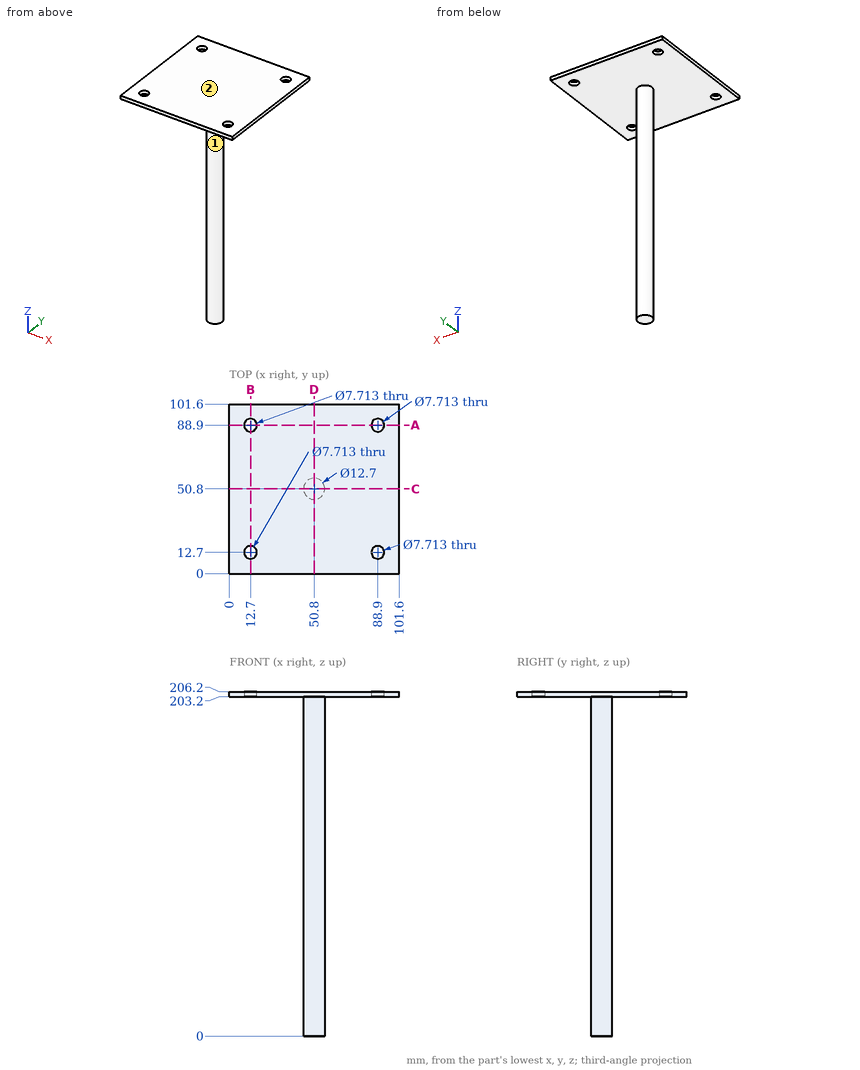
Input: dimensioned drawing with shaded views. Units: mm. Origin: part minimum x, y, z. Round coordinates to 2 decimals unless told otherwise and drop trailing zeros. Order: outer loops, then holes, each group sorted by start corner. A loop starts at its lowest first (then second) coordinate and runs counter-clockwise, first axis right, second up. Notation, with made-up numbers: (37, 22.25) -> (47, 22.25) arc R30 cw to (47, 49.25) -> close; hole circle Ø9 at (45.25, -18). An arc over 180 degrees is marked (long way). One line per item, written item: value. Start each with the question number.
Q1. Material intervals for probe 1 along Y at (x, z) = (12.7, 203.95); probe 2 along Y at (x, z) = (88, 204), sorted ascending.
Q2. Draft query along X for the marked faces 1 and 2. Return one class per face: pulls with the +X half, pulls with the -X half, needs draft (parallel to the pull), parting line crosses it, or undercut.
Q3. Section query A-A (y = 88.9). Return the cut outline in (x, z).
Q4. Section query C-C (y = 50.8). Return the cut outline in (x, z), plus the area to 3 significant figures.
Q5. Pin query (flat end, axial travel): pin 1 (3 mm diameter, centred on x = 77.5, y = 38.5, fed in from -Z); pin 2 (4.5 mm diameter, centred on x = 12.7, y = 12.7, fed in from +Z). Return the tip coordinate at first contact, or that it passes through.
Findings below:
1. probe 1: 0 to 8.84, 16.56 to 85.04, 92.76 to 101.6
1. probe 2: 0 to 8.95, 16.45 to 85.15, 92.65 to 101.6
2. face 1: parting line crosses it
2. face 2: needs draft
3. outline: (0, 203.2) -> (8.84, 203.2) -> (8.84, 206.2) -> (0, 206.2) -> close; (16.56, 203.2) -> (85.04, 203.2) -> (85.04, 206.2) -> (16.56, 206.2) -> close; (92.76, 203.2) -> (101.6, 203.2) -> (101.6, 206.2) -> (92.76, 206.2) -> close
4. outline: (0, 203.2) -> (44.45, 203.2) -> (44.45, 0) -> (57.15, 0) -> (57.15, 203.2) -> (101.6, 203.2) -> (101.6, 206.2) -> (0, 206.2) -> close
4. area: 2,890 mm²
5. pin 1: z = 203.2
5. pin 2: through
